Geometry check sheet. Reference: the model listing, model coordinates, mm. A direction names the side the tool comes from. Give positions to 0.01 mm unless a question says otherwise; leave off trailing zeros. Write each loop counter-clockwise with the first axis right and the second up, starting at its lowest first coordinate (ties: lowest second). Pieces come first, ordered by that corner, then holes. Notation, with made-up numbers: (-14, 35.25) - (-6, 35.25) arc R15 cw to (-6, 56.25) - close; hole circle Ø5 at (39, 66). An arc over 180 degrees is marked (long way). Use a Markdown table: item, result.
```python
from build123d import *

# Parameters (mm, degrees)
SKETCH140_R         = 11.5
SKETCH140_R_2       = 6.5
PAD054_DEPTH        = 2
SKETCH141_R         = 8.5
SKETCH141_R_2       = 6.5
PAD055_DEPTH        = 10
SKETCH142_W         = 3
SKETCH142_H         = 2
PAD056_DEPTH        = 10
REVOLUTION015_ANGLE = -180
REVOLUTION016_ANGLE = -180
FILLET_R            = 1
SKETCH171_R         = 8
SKETCH171_R_2       = 6.5
PAD068_DEPTH        = 8


with BuildPart() as part:
    # Sketch140 → Pad054 (new body)
    with BuildSketch(Plane.XY):
        Circle(SKETCH140_R)
        Circle(SKETCH140_R_2, mode=Mode.SUBTRACT)
    extrude(amount=PAD054_DEPTH)

    # Sketch141 (on Face4 of Pad054) → Pad055 (join)
    with BuildSketch(Plane.XY.offset(2)):
        Circle(SKETCH141_R)
        Circle(SKETCH141_R_2, mode=Mode.SUBTRACT)
    extrude(amount=PAD055_DEPTH)

    # Sketch142 (on Face2 of Pad055) → Pad056 (join)
    with BuildSketch(Plane(origin=(0, 0, 0), x_dir=(1, 0, 0), z_dir=(0, 0, -1))):
        with Locations((0, 7.5)):
            Rectangle(SKETCH142_W, SKETCH142_H)
        with Locations((0, -7.5)):
            Rectangle(SKETCH142_W, SKETCH142_H)
    extrude(amount=PAD056_DEPTH)

    # Sketch154 (on Face11 of Pad056) → Revolution015 (revolve)
    with BuildSketch(Plane.XZ.offset(8.5)):
        with BuildLine():
            ThreePointArc((0, -4.5), (1, -3.5), (0, -2.5))
            Line((0, -2.5), (0, -4.5))
        make_face()
    revolve(axis=Axis((0, -8.5, 0), (0, 0, 1)), revolution_arc=REVOLUTION015_ANGLE)

    # Sketch155 (on Face7 of Revolution015) → Revolution016 (revolve)
    with BuildSketch(Plane(origin=(0, 8.5, 0), x_dir=(-1, 0, 0), z_dir=(0, 1, 0))):
        with BuildLine():
            ThreePointArc((0, -4.5), (1, -3.5), (0, -2.5))
            Line((0, -2.5), (0, -4.5))
        make_face()
    revolve(axis=Axis((0, 8.5, 0), (0, 0, 1)), revolution_arc=REVOLUTION016_ANGLE)

    # Fillet
    fillet_edges = [part.edges().sort_by_distance(p)[0] for p in [
        (0, 8.5, -10),
        (0, -8.5, -10),
    ]]
    fillet(fillet_edges, radius=FILLET_R)

    # Sketch171 (on Face6 of Fillet) → Pad068 (join)
    with BuildSketch(Plane(origin=(0, 0, 0), x_dir=(1, 0, 0), z_dir=(0, 0, -1))):
        Circle(SKETCH171_R)
        Circle(SKETCH171_R_2, mode=Mode.SUBTRACT)
    extrude(amount=PAD068_DEPTH)


with BuildPart() as part_1:
    # Body placement: moved
    add(part.part.moved(Location((0, 0, -10))))


solid = part_1.part
```
1) Section check B-B on y = 0. Record the boundary of the cut face in (x, z).
Working result:
| item | result |
|---|---|
| outline | (-11.5, -10) - (-8, -10) - (-8, -18) - (-6.5, -18) - (-6.5, 2) - (-8.5, 2) - (-8.5, -8) - (-11.5, -8) - close; (6.5, -18) - (8, -18) - (8, -10) - (11.5, -10) - (11.5, -8) - (8.5, -8) - (8.5, 2) - (6.5, 2) - close |
2) Section check A-A on z = -13.5. Record the boundary of the cut face in (x, y).
Working result:
| item | result |
|---|---|
| outline | (-1.5, -8.5) - (-1, -8.5) arc R1 ccw to (1, -8.5) - (1.5, -8.5) - (1.5, -7.86) arc R8 ccw to (1.5, 7.86) - (1.5, 8.5) - (1, 8.5) arc R1 ccw to (-1, 8.5) - (-1.5, 8.5) - (-1.5, 7.86) arc R8 ccw to (-1.5, -7.86) - close; hole circle Ø13 at (0, 0) |
3) Set-up check for faces 1 (the cylindrical face through (8, 0, -14)), 2 (the flat face through (1.5, 8.2, -16)), 3 (the flat face through (-1.5, -8.2, -16)), 4 (the cylindrical face through (4.57, 7.167, -3.07)): record each of +Z, -Z, +X, -X, +Y, -Y from which the full face is reachable in a straight line by a thin tool's end or side.
Working result:
| item | result |
|---|---|
| face 1 | -Z, +X |
| face 2 | -Z, +X, +Y |
| face 3 | -Z, -X, -Y |
| face 4 | +Z |
4) Material ranges on L1, parallel to Y at x = 0, z = -11.5; L2, parallel to Z at x = 6.25, y = 6; L3, parallel to X at y = 8, z = -19, recorded low to high. Write a range as from..to.
Working result:
| item | result |
|---|---|
| L1 | y = -8.5..-6.5, 6.5..8.5 |
| L2 | z = -10..-8 |
| L3 | x = -1.5..1.5 |
5) Mould release check, pull along Z, two halves, no side actions. Record for faces 5 (the flat face through (-0.69, 8.5, -14.44)), 6 (the flat face through (-4, -8, -8)), 7 (the flat face through (0, 6.5, -19)), 8 (the flat face through (-0.69, -8.5, -14.44)): pulls with the +Z half, pulls with the -Z half, needs draft (parallel to the pull), parting line crosses it, or undercut.
Working result:
| item | result |
|---|---|
| face 5 | undercut |
| face 6 | pulls with the +Z half |
| face 7 | needs draft |
| face 8 | undercut |
6) Section check C-C on x = -5. Record the boundary of the cut face in (y, z) (3 decimals).
Working result:
| item | result |
|---|---|
| outline | (-10.356, -10) - (-6.245, -10) - (-6.245, -18) - (-4.153, -18) - (-4.153, 2) - (-6.874, 2) - (-6.874, -8) - (-10.356, -8) - close; (4.153, -18) - (6.245, -18) - (6.245, -10) - (10.356, -10) - (10.356, -8) - (6.874, -8) - (6.874, 2) - (4.153, 2) - close |
7) Depth check by flat-ended pin: P1, Ø1, axis at x = -1, z = -13.5, coming from the -Y side; P2, Ø4, axis at x = -9, z = -2, coming from the +Y side; P3, Ø1.6, axis at y = -7.5, z = -13, coming from the -X side; P4, Ø4, axis at x = -3, y = 0, coming from the -Z side. Enter the tip coordinate at first touch or a pass-through.
Working result:
| item | result |
|---|---|
| P1 | stops at y = -9.37 |
| P2 | stops at y = 4.82 |
| P3 | stops at x = -4.37 |
| P4 | passes through |
8) Section check D-D on z = -9. Record the boundary of the cut face in (x, y), then the cut area to 3 significant figures.
Working result:
| item | result |
|---|---|
| outline | circle Ø23 at (0, 0); hole circle Ø13 at (0, 0) |
| area | 283 mm² |
